CAD build for the part. Positions are in the model's coordinates, mm. Face numbers are marked on the shaded views. A direction names the side the tool comes from. Round coordinates to 2 decimals unless told otherwise and drop trailing zeros. Write each loop counter-clockwise with the first axis right and the second up, starting at its lowest first coordinate (ties: lowest second). Pieces come first, ordered by that corner, then holes. Notation, with made-up numbers: (14, 30) -> (54, 30) arc R19 ccw to (54, 63) -> close; hole circle Ø5 at (-31, 63). An arc over 180 degrees is marked (long way). Put each result on its own line as item: value. Start each with the question number.
1. Saw through at A-A on z = 1.5. List the corners of the cut face in (x, y).
2. Flat gauge pins, fed straight in: P1, Ø5, axis at y = 2.5, z = 7, coming from the +X side; P2, Ø4, axis at y = 5, z = 5.5, coming from the +X side; P3, Ø8, axis at x = 17, y = -7.5, coming from the +Z side. Where does each tip first touch, or does it go through?
3. Saw through at D-D on x = 6.75. List the corners of the cut face in (y, z), and give its area (3 significant figures).
4. Saw through at B-B on x = 9. List the corners of the cut face in (y, z).
5. Saw through at C-C on y = 0.5. List the corners of the cut face in (x, z).
6. 3-axis set-ups, long thin cutter, end or side, ignore diameter. For the marked faces 1, 2 and 3: which of +Z, -Z, +X, -X, +Y, -Y reach the whole face in a straight line?
7. Drill centre lines: line 1 (Z direction, x = 10.5, y = -7.25); line 2 (X direction, y = 4.75, z = 3.5); line 3 (Y direction, x = 13.25, z = 3.25). Where is each one in solid material? Low to high. Write a range as from..to.
from build123d import *

# Parameters (mm, degrees)
BOSS_EXTRUDE2_DEPTH = 10
SKETCH3_R           = 1.5
BOSS_EXTRUDE3_DEPTH = 2


with BuildPart() as part:
    # Sketch1 → Boss-Extrude2 (new body)
    with BuildSketch(Plane.XY):
        with BuildLine():
            Line((7.884962528, 10.248457422), (7.884962528, -2.471687197))
            ThreePointArc((7.884962528, -2.471687197), (7.318196318, -3.914788011), (6.259459635, -5.047413515))
            ThreePointArc((6.259459635, -5.047413515), (4.447305875, -7.175808801), (3.796141897, -9.894255639))
            Line((3.796141897, -9.894255639), (4.70457442, -9.894255639))
            ThreePointArc((4.70457442, -9.894255639), (7.134282097, -14.234596844), (12.104480976, -14.432496496))
            Line((12.104480976, -14.432496496), (13.766372841, -14.432496496))
            ThreePointArc((13.766372841, -14.432496496), (15.180586403, -13.846710058), (15.766372841, -12.432496496))
            Line((15.766372841, -12.432496496), (15.766372841, 5.828797616))
            ThreePointArc((15.766372841, 5.828797616), (16.123155433, 6.968901362), (17.066209392, 7.702235938))
            ThreePointArc((17.066209392, 7.702235938), (19.42011278, 11.840679713), (15.766372841, 14.893180737))
            Line((15.766372841, 14.893180737), (12.529685844, 14.893180737))
            ThreePointArc((12.529685844, 14.893180737), (9.245370491, 13.532772775), (7.884962528, 10.248457422))
        make_face()
    extrude(amount=BOSS_EXTRUDE2_DEPTH)

    # Sketch3 → Boss-Extrude3 (add)
    with BuildSketch(Plane.XY.offset(10)):
        with Locations((9.796141897, -9.894255639)):
            Circle(SKETCH3_R)
    extrude(amount=BOSS_EXTRUDE3_DEPTH)


solid = part.part
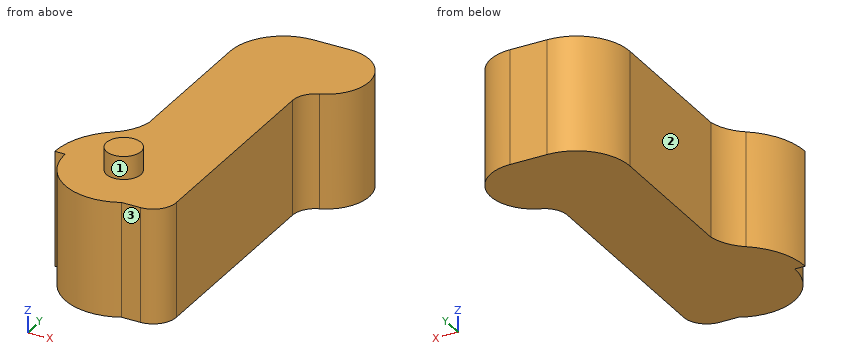
Return value:
1. outline: (3.8, -9.89) -> (4.7, -9.89) arc R5.09 ccw to (12.1, -14.43) -> (13.77, -14.43) arc R2 ccw to (15.77, -12.43) -> (15.77, 5.83) arc R2 cw to (17.07, 7.7) arc R3.71 ccw to (15.77, 14.89) -> (12.53, 14.89) arc R4.64 ccw to (7.88, 10.25) -> (7.88, -2.47) arc R4.13 cw to (6.26, -5.05) arc R6 ccw to start
2. P1: stops at x = 15.77
2. P2: stops at x = 16.15
2. P3: stops at z = 10
3. outline: (-13.97, 0) -> (-4.63, 0) -> (-4.63, 10) -> (-13.97, 10) -> close
3. area: 93.5 mm^2
4. outline: (-14.92, 0) -> (13.27, 0) -> (13.27, 10) -> (-8.62, 10) -> (-8.62, 12) -> (-11.17, 12) -> (-11.17, 10) -> (-14.92, 10) -> close
5. outline: (7.88, 0) -> (15.77, 0) -> (15.77, 10) -> (7.88, 10) -> close
6. face 1: +Z
6. face 2: +Z, -Z, -X, +Y
6. face 3: +Z, -Z, +X, -Y
7. line 1: z = 0..10
7. line 2: x = 7.88..15.77
7. line 3: y = -14.43..14.89
